```python
from build123d import *

# Parameters (mm, degrees)
BOSS_EXTRUDE1_DEPTH          = 8
SKETCH2_R                    = 4
CUT_EXTRUDE1_DEPTH           = 45
CUT_EXTRUDE1_TAPER           = 5
CUT_EXTRUDE1_OTHER_WAY_DEPTH = 1
SKETCH3_R                    = 2.1
BOSS_EXTRUDE2_DEPTH          = 3
FILLET1_R                    = 2
SKETCH4_R                    = 2.1
CUT_EXTRUDE2_DEPTH           = 16
FILLET1_OF_MIRROR1_R         = 2
SKETCH5_R                    = 2.85
CUT_EXTRUDE3_DEPTH           = 25.1


with BuildPart() as part:
    # Sketch1 → Boss-Extrude1 (new body, symmetric)
    with BuildSketch(Plane(origin=(0, 0, 0), x_dir=(0, 0, -1), z_dir=(1, 0, 0))):
        Polygon((-56.4, 122.940542206), (-56.4, 0), (-40.4, 0), (-40.4, 110), (0, 118.638335016), (40.4, 110), (40.4, 0), (56.4, 0), (56.4, 122.940542206), (0, 135), align=None)
    extrude(amount=BOSS_EXTRUDE1_DEPTH, both=True)

    # Sketch2 → Cut-Extrude1 (cut)
    with BuildSketch(Plane.XZ):
        with Locations((-8, -56.4)):
            Circle(SKETCH2_R)
        with Locations((8, -56.4)):
            Circle(SKETCH2_R)
    cut_extrude1 = extrude(amount=-CUT_EXTRUDE1_DEPTH, taper=CUT_EXTRUDE1_TAPER, mode=Mode.SUBTRACT)

    # Sketch2 → Cut-Extrude1 other way (cut)
    with BuildSketch(Plane.XZ):
        with Locations((-8, -56.4)):
            Circle(SKETCH2_R)
        with Locations((8, -56.4)):
            Circle(SKETCH2_R)
    extrude(amount=CUT_EXTRUDE1_OTHER_WAY_DEPTH, mode=Mode.SUBTRACT)

    # Sketch3 → Boss-Extrude2 (add)
    with BuildSketch(Plane(origin=(0, 0, 0), x_dir=(1, 0, 0), z_dir=(0, 1, 0))):
        Polygon((-8, 40.4), (8, 40.4), (16.1, 52.5), (16.1, 64.5), (-16.1, 64.5), (-16.1, 52.5), align=None)
        with Locations((-8, 56.4)):
            Circle(SKETCH3_R, mode=Mode.SUBTRACT)
        with Locations((8, 56.4)):
            Circle(SKETCH3_R, mode=Mode.SUBTRACT)
    boss_extrude2 = extrude(amount=BOSS_EXTRUDE2_DEPTH)

    # Fillet1
    fillet1_edges = [part.edges().sort_by_distance(p)[0] for p in [
        (16.1, 1.5, -52.5),
        (16.1, 1.5, -64.5),
        (-16.1, 1.5, -64.5),
        (-16.1, 1.5, -52.5),
    ]]
    fillet(fillet1_edges, radius=FILLET1_R)

    # Sketch4 → Cut-Extrude2 (cut)
    with BuildSketch(Plane(origin=(0, 0, -56.4), x_dir=(-1, 0, 0), z_dir=(0, 0, -1))):
        with Locations((0.9, 59)):
            Circle(SKETCH4_R)
        with Locations((0.9, 43)):
            Circle(SKETCH4_R)
    cut_extrude2 = extrude(amount=-CUT_EXTRUDE2_DEPTH, mode=Mode.SUBTRACT)

    # Mirror1: Cut-Extrude1, Boss-Extrude2, Cut-Extrude2 across plane
    add(cut_extrude1.mirror(Plane.XY), mode=Mode.SUBTRACT)
    add(boss_extrude2.mirror(Plane.XY))
    add(cut_extrude2.mirror(Plane.XY), mode=Mode.SUBTRACT)

    # Fillet1 of Mirror1
    fillet1_of_mirror1_edges = [part.edges().sort_by_distance(p)[0] for p in [
        (16.1, 1.5, 52.5),
        (16.1, 1.5, 64.5),
        (-16.1, 1.5, 64.5),
        (-16.1, 1.5, 52.5),
    ]]
    fillet(fillet1_of_mirror1_edges, radius=FILLET1_OF_MIRROR1_R)

    # Sketch5 → Cut-Extrude3 (cut, through all)
    with BuildSketch(Plane(origin=(8, 0, 0), x_dir=(0, 0, -1), z_dir=(1, 0, 0))):
        with Locations((0, 127)):
            Circle(SKETCH5_R)
    extrude(amount=-CUT_EXTRUDE3_DEPTH, mode=Mode.SUBTRACT)


solid = part.part
```
Input: part model. Units: mm. Frame: model coordinates. A direction names the side the tool comes from. Give positions to 0.01 mm unless a question says otherwise; leave off trailing zeros. Loops run counter-clockwise (first coordinate to the right, second up) from the corner with the lowest first, then second, coordinate; pieces in that order, holes last.
1) Line query: L1, parallel to X at y = 1.9, z = -56.4; L2, parallel to Y at x = -0.9, z = 52.5; L3, parallel to Z at x = 5, y = 19. Output: solid intervals per line, ascending.
A:
L1: x = -16.1 to -10.1, -5.9 to 5.9, 10.1 to 16.1
L2: y = 0 to 40.9, 45.1 to 56.9, 61.1 to 123.77
L3: z = -56.4 to -40.4, 40.4 to 56.4
2) Section query D-D on y = 127. Return the cut outline in (x, z).
A:
outline: (-8, -37.41) - (8, -37.41) - (8, -2.85) - (-8, -2.85) - close; (-8, 2.85) - (8, 2.85) - (8, 37.41) - (-8, 37.41) - close
3) Mould query, pull axis X, two halves, no side actions, for faces 1 (the flat face through (0, 56, -40.4)), 2 (the cylindrical face through (-0.44, 56.95, 48.51)), 3 (the flat face through (-16.1, 1, 58)). Classes: released by +X, released by -X, zero draft, split by the parting line, or undercut.
A:
face 1: zero draft
face 2: undercut
face 3: released by -X
4) Section query C-C on y = 43. Return the cut outline in (x, z), and give its area (3 significant figures).
A:
outline: (-8, -56.16) arc R0.24 cw to (-7.76, -56.4) - (-3, -56.4) - (-3, -40.4) - (-8, -40.4) - close; (-8, 40.4) - (-3, 40.4) - (-3, 56.4) - (-7.76, 56.4) arc R0.24 cw to (-8, 56.16) - close; (1.2, -56.4) - (7.76, -56.4) arc R0.24 cw to (8, -56.16) - (8, -40.4) - (1.2, -40.4) - close; (1.2, 40.4) - (8, 40.4) - (8, 56.16) arc R0.24 cw to (7.76, 56.4) - (1.2, 56.4) - close
area: 377 mm2
5) Contact query for flat-ended pins moving along their axis: pin 1 (8 mm diameter, centred on y = 24, z = -38, fed in from -X); pin 2 (3.5 mm diameter, centred on y = 127, z = 0, fed in from +X); pin 3 (13 mm diameter, centred on x = 2, y = 54.5, fed in from +Z); pin 4 (5 mm diameter, centred on x = -0.9, y = 59, fed in from -Z). Output: stop coordinate, or through.
A:
pin 1: stops at x = -8
pin 2: passes through
pin 3: stops at z = 56.4
pin 4: stops at z = -56.4
6) Section query A-A on y = 68. Return the cut outline in (x, z), and give its area (3 significant figures).
A:
outline: (-8, -56.4) - (8, -56.4) - (8, -40.4) - (-8, -40.4) - close; (-8, 40.4) - (8, 40.4) - (8, 56.4) - (-8, 56.4) - close
area: 512 mm2
7) Section query B-B on x = -0.5. Count the separate pieces of the cut face and the enclosed holes in it, and give its area (3 significant figures).
A:
separate pieces: 5
enclosed holes: 1
area: 5,070 mm2
8) Reachability of faces 4 (the flat face through (0, 54, 40.4)), 5 (the flat face through (-8, 118, 4)), 6 (the conical face through (-6.66, 24.29, 55.09)), 7 (the flat face through (11.83, 1.48, 46.12)), 8 (the conical face through (6.69, 24.29, -55.06)) from +Z, -Z, +X, -X, +Y, -Y: full face, straight path, thin tool, end or side. Return the list, or none.
A:
face 4: +X, -X, -Y
face 5: +Z, -Z, -X, +Y
face 6: +Z, -X
face 7: +X, +Y, -Y
face 8: -Z, +X
